Design review of the part built by this model. Coordinates are the model's own, in mm. A direction names the side the tool comes from. Coordinates: 2 decimals unless noted, no trailing zeros. Order: outer loops, then holes, each group sorted by start corner. A loop starts at its lowest first (then second) coordinate and runs counter-clockwise, first axis right, second up. Notation, with made-up numbers: M 25,21.5 L 71,21.5 A14 cw 71,26.5 Z; hole C 42.25,66.25 d9. An arc over 180 degrees is marked long. Answer in a Markdown table with one row per item.
from build123d import *

# Parameters (mm, degrees)
F0_W     = 101.6
F0_H     = 203.2
F1_DEPTH = 12.7
F2_W     = 101.6
F2_H     = 12.7
F3_DEPTH = 101.6
F5_D     = 19.05
F5_DEPTH = 12.7
F7_D     = 19.05
F7_DEPTH = 12.7
F9_D     = 19.05
F9_DEPTH = 12.7


with BuildPart() as f1:
    # F0 (on Front) → F1 (new body)
    with BuildSketch(Plane.XZ):
        with Locations((50.8, 101.6)):
            Rectangle(F0_W, F0_H)
    extrude(amount=F1_DEPTH)

    # F2 (on face) → F3 (join)
    with BuildSketch(Plane.XZ.offset(12.7)):
        with Locations((50.8, 6.35)):
            Rectangle(F2_W, F2_H)
    extrude(amount=F3_DEPTH)

    # F5
    with Locations(Plane.XY.offset(12.7)):
        with Locations((25.4, -88.9)):
            Hole(F5_D / 2, depth=F5_DEPTH)

    # F7
    with Locations(Plane.XY.offset(12.7)):
        with Locations((25.4, -38.1), (76.2, -38.1), (76.2, -88.9)):
            Hole(F7_D / 2, depth=F7_DEPTH)

    # F9
    with Locations(Plane.XZ.offset(12.7)):
        with Locations((25.4, 152.4), (76.2, 152.4), (76.2, 63.5), (25.4, 63.5)):
            Hole(F9_D / 2, depth=F9_DEPTH)


solid = f1.part
(1) Add section A-A, the plane y = -88.9. Give the boundary of the cut face in (x, z) (3 decimals).
Return value:
| item | result |
|---|---|
| outline | M 0,0 L 15.875,0 L 15.875,12.7 L 0,12.7 Z; M 34.925,0 L 66.675,0 L 66.675,12.7 L 34.925,12.7 Z; M 85.725,0 L 101.6,0 L 101.6,12.7 L 85.725,12.7 Z |
(2) Add section B-B, the plane x = 76.2. Give the boundary of the cut face in (y, z) (3 decimals).
Return value:
| item | result |
|---|---|
| outline | M -114.3,0 L -98.425,0 L -98.425,12.7 L -114.3,12.7 Z; M -79.375,0 L -47.625,0 L -47.625,12.7 L -79.375,12.7 Z; M -28.575,0 L 0,0 L 0,53.975 L -12.7,53.975 L -12.7,12.7 L -28.575,12.7 Z; M -12.7,73.025 L 0,73.025 L 0,142.875 L -12.7,142.875 Z; M -12.7,161.925 L 0,161.925 L 0,203.2 L -12.7,203.2 Z |
(3) Insertion check: pin 1 Ø10 at (x, z) = (43, 24) entering from -Y; pin 2 Ø15 at (x, z) = (25.4, 63.5) entering from +Y; pin 3 Ø12 at (x, y) = (52.5, -85.5) entering from +Z. Each pin has a flat end and moves straight along its axis. Give the tip position at first contact, or say it passes through.
Return value:
| item | result |
|---|---|
| pin 1 | stops at y = -12.7 |
| pin 2 | passes through |
| pin 3 | stops at z = 12.7 |
(4) Add section D-D, the plane x = 37. Give the boundary of the cut face in (y, z), and give its area (3 significant figures).
Return value:
| item | result |
|---|---|
| outline | M -114.3,0 L 0,0 L 0,203.2 L -12.7,203.2 L -12.7,12.7 L -114.3,12.7 Z |
| area | 3,870 mm2 |
(5) Draft analysis for pull direction Y (two halves, no side actions). For faces 3 (the flat face through (50, 0, 103)), 4 (the cylindrical face through (26.64, -6.261, 72.944)), 5 (the cylindrical face through (26.64, -79.456, 6.261)), state which applies: pulls with the +Y half, pulls with the -Y half, needs draft (parallel to the pull), parting line crosses it, or undercut.
Return value:
| item | result |
|---|---|
| face 3 | pulls with the +Y half |
| face 4 | needs draft |
| face 5 | undercut |
(6) For faces 1 (the flat face through (50, -12.7, 109)), 2 (the flat face through (50, -56, 0)), list the 3-axis set-ups (+Z, -Z, +X, -X, +Y, -Y) from which the entire face can be reached by the end or side of a thin tool; tool diameter is ignored.
Return value:
| item | result |
|---|---|
| face 1 | +Z, +X, -X, -Y |
| face 2 | -Z, +X, -X, +Y, -Y |
(7) For line 1 along Z through (x, y) = (25, -5); line 2 along X through (y, z) = (-9, 152); line 3 along Y through (x, z) = (25.4, 7.75) (3 decimals), list the stretches that pass through material, from the lowest coordinate up. Write a range as from..to.
Return value:
| item | result |
|---|---|
| line 1 | z = 0..53.98, 73.02..142.88, 161.92..203.2 |
| line 2 | x = 0..15.88, 34.92..66.68, 85.72..101.6 |
| line 3 | y = -114.3..-98.425, -79.375..-47.625, -28.575..0 |
(8) Add section C-C, the plane z = 63.5. Give the boundary of the cut face in (x, y) (3 decimals), and give its area (3 significant figures).
Return value:
| item | result |
|---|---|
| outline | M 0,-12.7 L 15.875,-12.7 L 15.875,0 L 0,0 Z; M 34.925,-12.7 L 66.675,-12.7 L 66.675,0 L 34.925,0 Z; M 85.725,-12.7 L 101.6,-12.7 L 101.6,0 L 85.725,0 Z |
| area | 806 mm2 |
